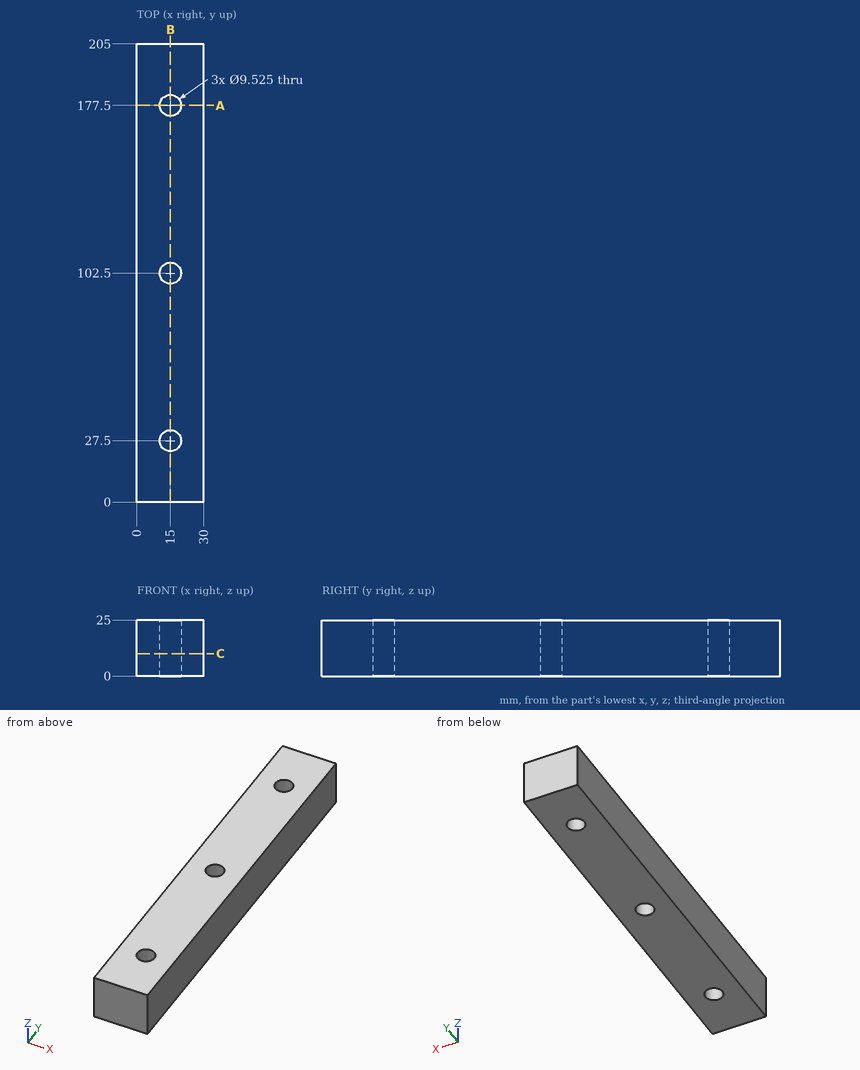
Source: three-view drawing plus pictorial views. Frame: mm from the lowest corner of the part. Give positions to 0.01 mm unless a question says otherwise; leave off trailing zeros. Order: outer loops, then holes, each group sorted by start corner. A loop starts at its lowest first (then second) coordinate and runs counter-clockwise, first axis right, second up. Notation, with made-up numbers: (25.5, 71.25) -> (79.5, 71.25) arc R24 ccw to (79.5, 106.25) -> close; hole circle Ø4 at (-13.5, 45.5). An arc over 180 degrees is marked (long way). Use a Markdown table: item, result.
Q1. Section A-A (y = 177.5). Return the cut outline in (x, z).
A:
| item | result |
|---|---|
| outline | (0, 0) -> (10.24, 0) -> (10.24, 25) -> (0, 25) -> close; (19.76, 0) -> (30, 0) -> (30, 25) -> (19.76, 25) -> close |
Q2. Section B-B (x = 15). Return the cut outline in (y, z).
A:
| item | result |
|---|---|
| outline | (0, 0) -> (22.74, 0) -> (22.74, 25) -> (0, 25) -> close; (32.26, 0) -> (97.74, 0) -> (97.74, 25) -> (32.26, 25) -> close; (107.26, 0) -> (172.74, 0) -> (172.74, 25) -> (107.26, 25) -> close; (182.26, 0) -> (205, 0) -> (205, 25) -> (182.26, 25) -> close |
Q3. Section C-C (z = 10). Return the cut outline in (x, y) (1 decimal), and give its area (3 significant figures).
A:
| item | result |
|---|---|
| outline | (0, 0) -> (30, 0) -> (30, 205) -> (0, 205) -> close; hole circle Ø9.5 at (15, 27.5); hole circle Ø9.5 at (15, 102.5); hole circle Ø9.5 at (15, 177.5) |
| area | 5,940 mm^2 |
Q4. Material intervals for line 1 (Y direction, x = 15, z = 5.5); line 2 (X direction, y = 102.5, z = 18.75); line 3 (Y direction, x = 15.75, z = 3.5), sorted ascending. Write a range as [from, to].
A:
| item | result |
|---|---|
| line 1 | [0, 22.74], [32.26, 97.74], [107.26, 172.74], [182.26, 205] |
| line 2 | [0, 10.24], [19.76, 30] |
| line 3 | [0, 22.8], [32.2, 97.8], [107.2, 172.8], [182.2, 205] |
